Part print with two shaded views. Sizes in mm from the minimum x, y, z corner. Coordinates: 2 decimals unless noted, no trailing zeros. Write each loop counter-clockwise with the first axis right and the second up, starting at its lowest first coordinate (ties: lowest second). Pieces come first, ordered by that corner, then holes.
Q1. Band-saw the part on D-D, the plane z = 0.7. Write the cut outline in (x, y) (1 decimal), plus the area to 3 significant figures.
Q2. Band-saw the part on C-C, the plane x = 6.75. Write the cut outline in (y, z).
Q3. Band-saw the part on A-A, the plane z = 1.65. Write the cut outline in (x, y), plus the area to 3 significant figures.
Q4. Pull direction Y, two halves, no side cores. Call the marked faces 1 and 2: released by +Y, released by -Y, zero draft, split by the parting line, or undercut.
Q5. Band-saw the part on B-B, the plane y = 7.25. Write the cut outline in (x, z).
Q6. Pin check, flat tips, straight feed: P1, Ø1.1, axis at y = 11, z = 0.5, coming from the -X side; P2, Ø3, axis at x = 7.5, y = 1.5, coming from the -Z side; P3, Ø1.1, axis at x = 10, z = 1.5, coming from the +Y side; P4, Ø0.8, axis at x = 6, z = 1.5, coming from the -Y side. Stop position of each tip, or through.
Q7. Drill centre lines: probe 1 along Z at (x, y) = (13.5, 5); probe 2 along X at (y, z) = (5.75, 1.9); probe 3 along Y at (x, z) = (12.25, 0.7). Where is each one in solid material? Low to high.
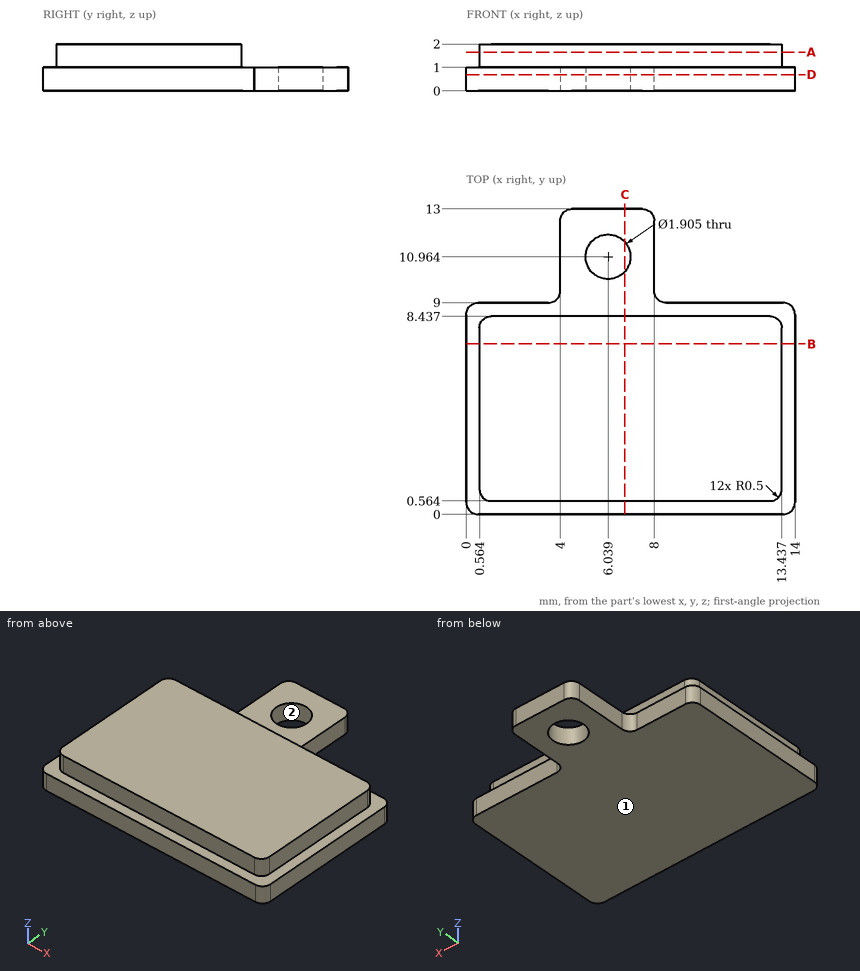
Answer sheet:
1. outline: (0, 0.5) arc R0.5 ccw to (0.5, 0) - (13.5, 0) arc R0.5 ccw to (14, 0.5) - (14, 8.5) arc R0.5 ccw to (13.5, 9) - (8.5, 9) arc R0.5 cw to (8, 9.5) - (8, 12.5) arc R0.5 ccw to (7.5, 13) - (4.5, 13) arc R0.5 ccw to (4, 12.5) - (4, 9.5) arc R0.5 cw to (3.5, 9) - (0.5, 9) arc R0.5 ccw to (0, 8.5) - close; hole circle Ø1.9 at (6, 11)
1. area: 139 mm2
2. outline: (0, 0) - (10.33, 0) - (10.33, 1) - (8.44, 1) - (8.44, 2) - (0.56, 2) - (0.56, 1) - (0, 1) - close; (11.6, 0) - (13, 0) - (13, 1) - (11.6, 1) - close
3. outline: (0.56, 1.06) arc R0.5 ccw to (1.06, 0.56) - (12.94, 0.56) arc R0.5 ccw to (13.44, 1.06) - (13.44, 7.94) arc R0.5 ccw to (12.94, 8.44) - (1.06, 8.44) arc R0.5 ccw to (0.56, 7.94) - close
3. area: 101 mm2
4. face 1: zero draft
4. face 2: undercut
5. outline: (0, 0) - (14, 0) - (14, 1) - (13.44, 1) - (13.44, 2) - (0.56, 2) - (0.56, 1) - (0, 1) - close
6. P1: stops at x = 4
6. P2: stops at z = 0
6. P3: stops at y = 9
6. P4: stops at y = 0.56
7. probe 1: z = 0 to 1
7. probe 2: x = 0.56 to 13.44
7. probe 3: y = 0 to 9
